Work out the finished part from the listing and answer in its coordinate system (mm). Face numbers are marked on the shaded views. A direction names the side the tool comes from. Give positions to 0.01 mm unless a question says otherwise; leave off trailing zeros. Loops run counter-clockwise (first coordinate to the right, second up) from the corner with the lowest first, then second, coordinate; pieces in that order, holes last. Notation, with made-up numbers: (21.25, 66.5) - (51.25, 66.5) arc R20 cw to (51.25, 98.5) - close; hole circle Ø2 at (25, -3.75). An arc over 180 degrees is marked (long way). One line per item, written item: value.
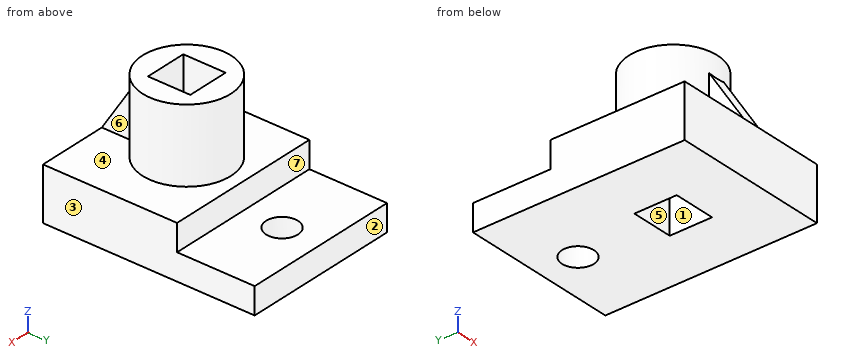
from build123d import *

# Parameters (mm, degrees)
SKETCH_1_W          = 45
SKETCH_1_H          = 60
EXTRUDE_1_DEPTH     = 15
SKETCH_2_W          = 7.5
SKETCH_2_H          = 22
CUT_EXTRUDE_1_DEPTH = 57.124860802
SKETCH_3_R          = 12.5
EXTRUDE_2_DEPTH     = 21
SKETCH_6_R          = 4.5
CUT_EXTRUDE_4_DEPTH = 48.100955404
RIB_1_REACH         = 53.983
SKETCH_7_WALL_W     = 123.721621612
SKETCH_7_WALL_H     = 5
SKETCH_8_W          = 12
SKETCH_8_H          = 12
CUT_EXTRUDE_5_DEPTH = 52.983170353


with BuildPart() as part:
    # Эскиз1 → Бобышка-Вытянуть1 (new body)
    with BuildSketch(Plane.XY):
        Rectangle(SKETCH_1_W, SKETCH_1_H)
    extrude(amount=EXTRUDE_1_DEPTH)

    # Эскиз2 → Вырез-Вытянуть1 (cut, through all)
    with BuildSketch(Plane(origin=(22.5, 0, 0), x_dir=(0, 0, -1), z_dir=(1, 0, 0))):
        with Locations((-11.25, 19)):
            Rectangle(SKETCH_2_W, SKETCH_2_H)
    extrude(amount=-CUT_EXTRUDE_1_DEPTH, mode=Mode.SUBTRACT)

    # Эскиз3 → Бобышка-Вытянуть2 (add)
    with BuildSketch(Plane.XY.offset(15)):
        with Locations(Location((0, -8, 0), (0, 0, 180))):
            Circle(SKETCH_3_R)
    extrude(amount=EXTRUDE_2_DEPTH)

    # Эскиз6 → Вырез-Вытянуть4 (cut, through all)
    with BuildSketch(Plane.XY.offset(7.5)):
        with Locations((0, 19)):
            Circle(SKETCH_6_R)
    extrude(amount=-CUT_EXTRUDE_4_DEPTH, mode=Mode.SUBTRACT)

    # Эскиз7 wall → Ребро1 (add, up to next)
    with BuildSketch(Plane(origin=(0, -25.25, 22.5), x_dir=(0, -0.535052081184, -0.844819075554), z_dir=(0, 0.844819075554, -0.535052081184)), mode=Mode.PRIVATE) as rib_1_sk1:
        Rectangle(SKETCH_7_WALL_W, SKETCH_7_WALL_H)
    rib_1_tool1 = extrude(rib_1_sk1.sketch, amount=RIB_1_REACH, mode=Mode.PRIVATE) - part.part
    add(rib_1_tool1.solids().sort_by_distance((0, -25.25, 22.5))[0])

    # Эскиз8 → Вырез-Вытянуть5 (cut, through all)
    with BuildSketch(Plane.XY.offset(36)):
        with Locations((0, -8)):
            Rectangle(SKETCH_8_W, SKETCH_8_H)
    extrude(amount=-CUT_EXTRUDE_5_DEPTH, mode=Mode.SUBTRACT)


solid = part.part
1. Section A-A (x = 0) is taken. Write down the section's boundary in (y, z), and give its area (3 significant figures).
Output:
outline: (-30, 0) - (-14, 0) - (-14, 36) - (-20.5, 36) - (-20.5, 30) - (-30, 15) - close; (-2, 0) - (14.5, 0) - (14.5, 7.5) - (8, 7.5) - (8, 15) - (4.5, 15) - (4.5, 36) - (-2, 36) - close; (23.5, 0) - (30, 0) - (30, 7.5) - (23.5, 7.5) - close
area: 832 mm²
2. Section B-B (y = 19) is taken. Write down the section's boundary in (x, z), and give its area (3 significant figures).
Output:
outline: (-22.5, 0) - (-4.5, 0) - (-4.5, 7.5) - (-22.5, 7.5) - close; (4.5, 0) - (22.5, 0) - (22.5, 7.5) - (4.5, 7.5) - close
area: 270 mm²
3. Flat-ended cylindrical pins translate along their axes: pin 1 Ø3 at (x, z) = (18, 16) entering from +Y; pin 2 Ø12 at (x, z) = (-10.5, 29) entering from +Y; pin 3 Ø5 at (y, z) = (-24, 26) entering from +X. Find the tip coordinate at first contact, or state that the pin passes through.
Output:
pin 1: stops at y = 8
pin 2: stops at y = 3.66
pin 3: stops at x = 2.5
4. Section C-C (z = 28.5) is taken. Write down the section's boundary in (x, y).
Output:
outline: (-2.5, -21.45) - (2.5, -21.45) - (2.5, -20.25) arc R12.5 ccw (long way) to (-2.5, -20.25) - close; hole (-6, -14) - (6, -14) - (6, -2) - (-6, -2) - close
5. For the marked faces 4, 5, 6 and 7, determine the directions among +Z, -Z, +X, -X, +Y, -Y from which every point of the face is accessible in a straight line to the end or side of a thin tool.
Output:
face 4: +Z
face 5: +Z, -Z
face 6: +Z, +X, -Y
face 7: +Z, +X, -X, +Y
6. The mould has two halves that part along Y. Classify the marked faces 1, 2 and 3: released by +Y, released by -Y, zero draft, split by the parting line, or undercut.
Output:
face 1: undercut
face 2: released by +Y
face 3: zero draft
7. Find the intervals of material crossed by line 1 along Y through (x, z) = (0, 4); line 2 along X through (y, z) = (-7.5, 11); line 3 along Z through (x, y) = (10, 16.5), in increasing order.
Output:
line 1: y = -30 to -14, -2 to 14.5, 23.5 to 30
line 2: x = -22.5 to -6, 6 to 22.5
line 3: z = 0 to 7.5
8. Section D-D (y = -11.5) is taken. Write down the section's boundary in (x, z), and give its area (3 significant figures).
Output:
outline: (-22.5, 0) - (-6, 0) - (-6, 36) - (-12, 36) - (-12, 15) - (-22.5, 15) - close; (6, 0) - (22.5, 0) - (22.5, 15) - (12, 15) - (12, 36) - (6, 36) - close
area: 747 mm²
